from build123d import *

# Parameters (mm, degrees)
F1_DEPTH = 50.8
F0_W     = 7.62
F0_H     = 19.05
F2_DEPTH = 9.525
F3_R     = 6.35
F4_R     = 9.525
F5_DEPTH = 25.4
F6_DEPTH = 12.7


with BuildPart() as f1:
    # F0 (on Right) → F1 (new body, symmetric)
    with BuildSketch(Plane.YZ):
        Polygon((0, 63.5), (0, 0), (7.62, 0), (19.05, 0), (19.05, 63.5), align=None)
    extrude(amount=F1_DEPTH, both=True)

    # F0 (on Right) → F2 (join, symmetric)
    with BuildSketch(Plane.YZ):
        Polygon((0, 63.5), (0, 0), (7.62, 0), (19.05, 0), (19.05, 63.5), align=None)
        with Locations((3.81, -9.525)):
            Rectangle(F0_W, F0_H)
        with BuildLine():
            Line((7.62, -19.05), (0, -19.05))
            ThreePointArc((0, -19.05), (-25.016468, -50.077762), (-60.643908, -32.21072))
            Line((-60.643908, -32.21072), (-68.901188, -32.0802))
            ThreePointArc((-68.901188, -32.0802), (-25.141119, -57.861333), (7.62, -19.05))
        make_face()
    extrude(amount=F2_DEPTH, both=True)

    # F3
    f3_edges = [f1.edges().sort_by_distance(p)[0] for p in [
        (9.525, -64.772548, -32.14546),
        (-9.525, -64.772548, -32.14546),
        (50.8, 9.525, 0),
        (50.8, 9.525, 63.5),
        (-50.8, 9.525, 63.5),
        (-50.8, 9.525, 0),
    ]]
    fillet(f3_edges, radius=F3_R)

    # F4 (on face) → F5 (cut)
    with BuildSketch(Plane.XZ):
        with Locations((-30.197322, 44.45)):
            Circle(F4_R)
        with BuildLine():
            ThreePointArc((35.850874, 44.45), (26.325874, 53.975), (16.800874, 44.45))
            ThreePointArc((16.800874, 44.45), (26.325874, 34.925), (35.850874, 44.45))
        make_face()
    extrude(amount=-F5_DEPTH, mode=Mode.SUBTRACT)

    # F4 (on face) → F6 (cut)
    with BuildSketch(Plane.XZ):
        with Locations((-30.197322, 44.45)):
            Circle(F4_R)
        with BuildLine():
            ThreePointArc((35.850874, 44.45), (26.325874, 53.975), (16.800874, 44.45))
            ThreePointArc((16.800874, 44.45), (26.325874, 34.925), (35.850874, 44.45))
        make_face()
        with Locations((0, 19.05)):
            Circle(F4_R)
    extrude(amount=-F6_DEPTH, mode=Mode.SUBTRACT)


solid = f1.part
Could you check a few things on this model? Use its own coordinates, in mm. A direction names the side the tool comes from. Give positions to 0.01 mm unless a question says otherwise; leave off trailing zeros. Order: outer loops, then holes, each group sorted by start corner. A loop starts at its lowest first (then second) coordinate and runs counter-clockwise, first axis right, second up.
1. Suppose I cut it at C-C (z = -46). List the corners of the cut face in (x, y) for me (3 decimals).
2. We'd pull the mould along X, two halves only. Please class faces 5 (the cylindrical face through (-7.615, -64.251, -33.965)), 6 (the flat face through (50.8, 9, 32)), 7 (the cylindrical face through (-37.218, 9.392, 50.887)), 8 (the flat face through (1, 9, 0)): pulls with the +X half, pulls with the -X half, needs draft (parallel to the pull), parting line crosses it, or undercut.
3. I need wall thicknesses on L1, parallel to X at y = 4, z = 44; L2, parallel to X at y = 10, z = 19; L3, parallel to Y at x = -7.5, z = 49. Which ranges of each line are inside material? Lowest first, please.
4. Suppose I cut it at B-B (x = -34). List the corners of the cut face in (y, z) for me, plus the area to 3 significant figures.
5. Suppose I cut it at D-D (x = 0). List the corners of the cut face in (y, z) for me (3 decimals).
6. Will these pins go through, and if not, where does the flat tip stop? P1, Ø25, axis at x = 26.33, z = 44.45, coming from the -Y side; P2, Ø15, axis at x = -5, y = 9.5, coming from the -Z side; P3, Ø9.5, axis at x = -3.5, z = -7, coming from the +Y side; P4, Ø3, axis at y = -9, z = -37.5, coming from the -X side.
7. Suppose I cut it at A-A (z = 44.45). List the corners of the cut face in (x, y) for me.
8. For faces 1 (the flat face through (-9.525, -18, -49)), 2 (the flat face through (1, 0, 32)), 3 (the flat face through (9.525, -18, -49)), 4 (the cylindrical face through (-2.06, 6.26, 9.75)), which set-ups out of +Z, -Z, +X, -X, +Y, -Y let a thin tool reach every point of the face, with its end or its side?
Solved:
1. outline: (-9.525, -60.45) - (9.525, -60.45) - (9.525, -48.536) - (-9.525, -48.536) - close; (-9.525, -14.964) - (9.525, -14.964) - (9.525, -3.05) - (-9.525, -3.05) - close
2. face 5: pulls with the -X half
2. face 6: pulls with the +X half
2. face 7: undercut
2. face 8: needs draft
3. L1: x = -50.8 to -39.71, -20.68 to 16.81, 35.84 to 50.8
3. L2: x = -50.8 to -9.52, 9.52 to 50.8
3. L3: y = 0 to 19.05
4. outline: (0, 0) - (19.05, 0) - (19.05, 35.72) - (0, 35.72) - close; (0, 53.18) - (19.05, 53.18) - (19.05, 63.5) - (0, 63.5) - close
4. area: 877 mm2
5. outline: (-68.901, -32.08) arc R39.37 ccw to (7.62, -19.05) - (7.62, 0) - (19.05, 0) - (19.05, 63.5) - (0, 63.5) - (0, 28.575) - (12.7, 28.575) - (12.7, 9.525) - (0, 9.525) - (0, -19.05) arc R31.75 cw to (-60.644, -32.211) - close
6. P1: stops at y = 0
6. P2: stops at z = -39.32
6. P3: stops at y = 7.62
6. P4: passes through
7. outline: (-50.8, 0) - (-39.72, 0) - (-39.72, 19.05) - (-50.8, 19.05) - close; (-20.67, 0) - (16.8, 0) - (16.8, 19.05) - (-20.67, 19.05) - close; (35.85, 0) - (50.8, 0) - (50.8, 19.05) - (35.85, 19.05) - close
8. face 1: -Z, -X, +Y, -Y
8. face 2: +Z, +X, -X, -Y
8. face 3: -Z, +X, +Y, -Y
8. face 4: -Y
